For this review, take the finished solid that the model builds, in its own axes (mm). A direction names the side the tool comes from. Give positions to 0.01 mm unless a question says otherwise; leave off trailing zeros. Order: outer loops, then holes, each group sorted by start corner. A loop starts at its lowest first (then second) coordinate and runs counter-clockwise, first axis right, second up. Notation, with made-up numbers: (-28.5, -19) -> (-24.5, -19) arc R25 cw to (-24.5, 5) -> close; hole circle Ø3 at (-1.75, 7.25). An arc over 180 degrees is marked (long way). Return JSON: item names as keys, results as strings. Group by question number.
1) For faces 5 (the face through (31.75, 3, -14)), 6 (the face through (0, 0, -10)), 7 (the face through (0, 6.35, -12)), list the 3-axis set-ups (+Z, -Z, +X, -X, +Y, -Y) from which the entire face can be reached by the end or side of a thin tool; tool diameter is ignored.
2) To check wall thickness, follow line 1 along X through (y, z) = (-7.25, 1); line 2 along X through (y, z) = (5.75, -13); line 3 along Z through (x, y) = (-6.5, -4.75). State the ranges of each line that lie inside material, in increasing order.
3) The part is to be moulded in two halves that separate along Z. For faces 1 (the face through (-32.514, 3.519, -0.724)), 2 (the face through (-6.605, 3.131, -7.815)), 3 (the face through (9.192, 3.131, -5.733)), 4 (the face through (-1, 12.7, 1)), say which applies: released by +Z, released by -Z, zero draft, split by the parting line, or undercut.
4) Add section B-B (x = -36). Give the boundary of the cut face in (y, z), then the cut area to 3 significant figures.
5) Add section C-C (z = -4.25). Give the boundary of the cut face in (x, y), then the cut area to 3 significant figures.
6) Insertion check: P1, Ø6, axis at x = -37.36, y = -6.35, coming from the -Z side; P2, Ø4, axis at x = 0.5, z = -14.5, coming from the +Y side; P3, Ø10, axis at y = -4, z = -17, coming from the -X side. Each pin has a flat end and moves straight along its axis. Give the tip position at first contact, or say it passes through.
7) Add section A-A (y = -6.35). Give the boundary of the cut face in (x, z), then the cut area to 3 significant figures.
8) Add section D-D (x = 25.5). Give the boundary of the cut face in (y, z), then the cut area to 3 significant figures.
from build123d import *

# Parameters (mm, degrees)
SKETCH1_W           = 88.9
SKETCH1_H           = 25.4
BOSS_EXTRUDE1_DEPTH = 2.54
SKETCH2_R           = 2.032
SKETCH2_R_2         = 1.905
BOSS_EXTRUDE2_DEPTH = 6.35
SKETCH3_R           = 2.38125
CUT_EXTRUDE1_DEPTH  = 53.761321688
FILLET1_R           = 2.54


with BuildPart() as part:
    # Sketch1 → Boss-Extrude1 (new body)
    with BuildSketch(Plane.XY):
        Rectangle(SKETCH1_W, SKETCH1_H)
    extrude(amount=BOSS_EXTRUDE1_DEPTH)

    # Sketch2 → Boss-Extrude2 (add)
    with BuildSketch(Plane(origin=(0, 0, 0), x_dir=(1, 0, 0), z_dir=(0, 1, 0))):
        with BuildLine():
            Line((-31.75, 0), (-31.75, 25.429600199))
            ThreePointArc((-31.75, 25.429600199), (0, 15.8115), (31.75, 25.429600199))
            Line((31.75, 25.429600199), (31.75, 0))
            Line((31.75, 0), (0, 0))
            Line((0, 0), (-31.75, 0))
        make_face()
        with Locations(Location((-8.619949734, 7.549981355, 0), (0, 0, 270))):
            Circle(SKETCH2_R, mode=Mode.SUBTRACT)
        with Locations(Location((8.619949734, 7.549981355, 0), (0, 0, 270))):
            Circle(SKETCH2_R_2, mode=Mode.SUBTRACT)
    extrude(amount=BOSS_EXTRUDE2_DEPTH)

    # Sketch3 → Cut-Extrude1 (cut, through all)
    with BuildSketch(Plane(origin=(0, 0, 0), x_dir=(-1, 0, 0), z_dir=(0, 0, -1))):
        with Locations((-38.838399738, -6.35)):
            Circle(SKETCH3_R)
        with Locations((-0.738399738, -6.35)):
            Circle(SKETCH3_R)
        with Locations((37.361600262, -6.35)):
            Circle(SKETCH3_R)
    extrude(amount=-CUT_EXTRUDE1_DEPTH, mode=Mode.SUBTRACT)

    # Fillet1
    fillet1_edges = [part.edges().sort_by_distance(p)[0] for p in [
        (0, 6.35, 0),
        (31.75, 3.175, 0),
        (-31.75, 3.175, 0),
        (44.45, -12.7, 1.27),
        (-44.45, -12.7, 1.27),
        (-44.45, 12.7, 1.27),
        (44.45, 12.7, 1.27),
    ]]
    fillet(fillet1_edges, radius=FILLET1_R)


solid = part.part
Evaluation:
{
 "1": {"face 5": "-Z, +X, +Y, -Y", "face 6": "-Z, +X, -X, -Y", "face 7": "-Z, +X, -X, +Y"},
 "2": {"line 1": "-44.45 to -39.57, -35.16 to -1.47, 2.94 to 36.63, 41.04 to 44.45", "line 2": "-31.75 to 31.75", "line 3": "0 to 2.54"},
 "3": {"face 1": "released by -Z", "face 2": "undercut", "face 3": "undercut", "face 4": "zero draft"},
 "4": {"outline": "(-12.7, 0) -> (-8.3, 0) -> (-8.3, 2.54) -> (-12.7, 2.54) -> close; (-4.4, 0) -> (12.7, 0) -> (12.7, 2.54) -> (-4.4, 2.54) -> close", "area": "54.6 mm^2"},
 "5": {"outline": "(-31.75, 0) -> (31.75, 0) -> (31.75, 6.35) -> (-31.75, 6.35) -> close", "area": "403 mm^2"},
 "6": {"P1": "z = 0", "P2": "y = 6.35", "P3": "x = -31.75"},
 "7": {"outline": "(-44.45, 0) -> (-39.74, 0) -> (-39.74, 2.54) -> (-44.45, 2.54) -> close; (-34.98, 0) -> (-1.64, 0) -> (-1.64, 2.54) -> (-34.98, 2.54) -> close; (3.12, 0) -> (36.46, 0) -> (36.46, 2.54) -> (3.12, 2.54) -> close; (41.22, 0) -> (44.45, 0) -> (44.45, 2.54) -> (41.22, 2.54) -> close", "area": "190 mm^2"},
 "8": {"outline": "(-12.7, 0) -> (0, 0) -> (0, -21.81) -> (6.35, -21.81) -> (6.35, -2.54) arc R2.54 cw to (8.89, 0) -> (12.7, 0) -> (12.7, 2.54) -> (-12.7, 2.54) -> close", "area": "204 mm^2"}
}
